The model under review builds one solid part; all positions refer to its coordinate system, in mm. Face numbers are marked on the shaded views. A direction names the side the tool comes from. Coordinates: 2 decimals unless noted, no trailing zeros. Order: outer loops, then holes, each group sorted by start corner. A loop starts at its lowest first (then second) coordinate and runs counter-clockwise, first axis right, second up. Notation, with made-up numbers: M -10,89.25 L 34,89.25 A18 cw 34,105.25 Z; hole C 6.25,-21.75 d3. An arc over 180 degrees is marked long. Answer in a Markdown table with one row per item.
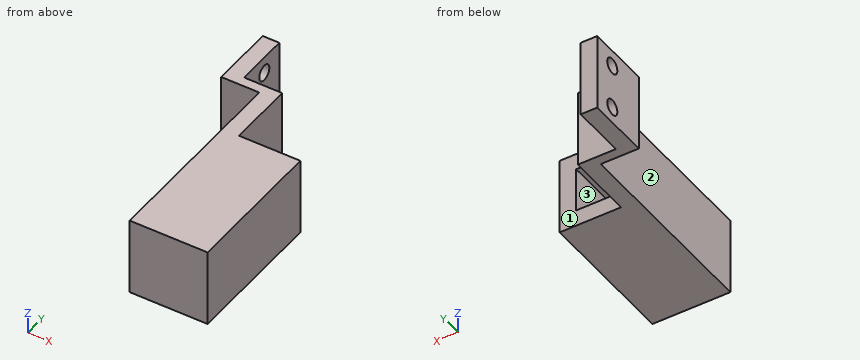
from build123d import *

# Parameters (mm, degrees)
BOSS_EXTRUDE1_DEPTH = 17.4
SKETCH3_W           = 10
SKETCH3_H           = 3.7
BOSS_EXTRUDE3_DEPTH = 30
SKETCH4_R           = 1.75
CUT_EXTRUDE1_DEPTH  = 55.985816353


with BuildPart() as part:
    # Sketch2 → Boss-Extrude1 (new body)
    with BuildSketch(Plane.XY):
        Polygon((-12.2, 12.2), (-8.5, 12.2), (-8.5, 0), (0, 0), (0, -45), (10, -45), (10, -15), (13.7, -15), (13.7, -47.2), (-3.7, -47.2), (-3.7, -2.2), (-12.2, -2.2), align=None)
    extrude(amount=BOSS_EXTRUDE1_DEPTH)

    # Sketch3 → Boss-Extrude3 (add)
    with BuildSketch(Plane.XZ.offset(45)):
        with Locations((5, 15.55)):
            Rectangle(SKETCH3_W, SKETCH3_H)
        with Locations((5, 1.85)):
            Rectangle(SKETCH3_W, SKETCH3_H)
    extrude(amount=-BOSS_EXTRUDE3_DEPTH)

    # Sketch4 → Cut-Extrude1 (cut, through all)
    with BuildSketch(Plane(origin=(-8.5, 0, 0), x_dir=(0, 0, -1), z_dir=(1, 0, 0))):
        with Locations((-13.7, 7)):
            Circle(SKETCH4_R)
        with Locations((-3.7, 7)):
            Circle(SKETCH4_R)
    extrude(amount=-CUT_EXTRUDE1_DEPTH, mode=Mode.SUBTRACT)


solid = part.part
(1) Take a section at B-B (z = 8). Write out the cut boundary in (x, y), then the cut area to 3 significant figures.
Report:
| item | result |
|---|---|
| outline | M -12.2,-2.2 L -3.7,-2.2 L -3.7,-47.2 L 13.7,-47.2 L 13.7,-15 L 10,-15 L 10,-45 L 0,-45 L 0,0 L -8.5,0 L -8.5,12.2 L -12.2,12.2 Z |
| area | 380 mm^2 |
(2) Machinability: for the marked faces 1, 2 and 3, which of the approach directions +Z, -Z, +X, -X, +Y, -Y give a long, thin tool a straight path to every point of the face, cutting with its end or side? Answer none if there is none.
Report:
| item | result |
|---|---|
| face 1 | +Z, -Z, +X, +Y |
| face 2 | +Z, -Z, -X, -Y |
| face 3 | +Y |
(3) Take a section at A-A (x = -9.25). Write out the cut boundary in (y, z), then the cut area to 3 significant figures.
Report:
| item | result |
|---|---|
| outline | M -2.2,0 L 12.2,0 L 12.2,17.4 L -2.2,17.4 Z; hole C 7,3.7 d3.5; hole C 7,13.7 d3.5 |
| area | 231 mm^2 |
(4) Take a section at C-C (y = -21.5). Write out the cut boundary in (x, z).
Report:
| item | result |
|---|---|
| outline | M -3.7,0 L 13.7,0 L 13.7,17.4 L -3.7,17.4 Z; hole M 0,3.7 L 10,3.7 L 10,13.7 L 0,13.7 Z |
(5) Insertion check: P1, Ø1.5, axis at x = 5.5, z = 10, coming from the +Y side; P2, Ø3, axis at y = 7, z = 13.7, coming from the +X side; P3, Ø6, axis at y = -4, z = 6, coming from the +X side; P4, Ø3, axis at y = -28, z = 7, coming from the -X side. Each pin has a flat end and moves straight along its axis. Give the tip position at first contact, or say it passes through.
Report:
| item | result |
|---|---|
| P1 | y = -45 |
| P2 | through |
| P3 | x = 0 |
| P4 | x = -3.7 |
(6) To check wall thickness, follow line 1 (X direction, y = -18, z = 7.5); line 2 (X direction, y = -10.5, z = 4); line 3 (Y direction, x = -11.2, z = 13.7). State the ranges of each line that lie inside material, in increasing order. Write a range as [from, to].
Report:
| item | result |
|---|---|
| line 1 | [-3.7, 0], [10, 13.7] |
| line 2 | [-3.7, 0] |
| line 3 | [-2.2, 5.25], [8.75, 12.2] |
(7) Take a section at D-D (y = 7). Write out the cut boundary in (x, z).
Report:
| item | result |
|---|---|
| outline | M -12.2,0 L -8.5,0 L -8.5,1.95 L -12.2,1.95 Z; M -12.2,5.45 L -8.5,5.45 L -8.5,11.95 L -12.2,11.95 Z; M -12.2,15.45 L -8.5,15.45 L -8.5,17.4 L -12.2,17.4 Z |
